For this review, take the finished solid that the model builds, in its own axes (mm). Coordinates: 2 decimals unless noted, no trailing zeros. Write each loop counter-clockwise with the first axis right and the second up, starting at its lowest first coordinate (ties: lowest second). Pieces come first, ordered by that corner, then holes. Notation, with made-up numbers: M -18,56.5 L 35,56.5 A16 cw 35,80.5 Z; hole C 79,47 d5. An arc over 180 degrees is marked long. Return JSON: item names as keys, results as strings.
```python
from build123d import *

# Parameters (mm, degrees)
SKETCH1_R = 25.4


with BuildPart() as part:
    # Sweep1: sweep along a curve in space
    with BuildLine() as sweep1_path:
        Line((0, 36.968559092, 0), (0, 36.968559092, -76.2))
        ThreePointArc((0, 36.968559092, -76.2), (0, 22.089583576, -112.121024484), (0, -13.831440908, -127))
        Line((0, -13.831440908, -127), (0, -217.031440908, -127))
        ThreePointArc((0, -217.031440908, -127), (0, -252.952465392, -112.121024484), (0, -267.831440908, -76.2))
        Line((0, -267.831440908, -76.2), (0, -267.831440908, -1.63913495))
        Line((0, -267.831440908, -1.63913495), (0, -267.831440908, 76.2))
        ThreePointArc((0, -267.831440908, 76.2), (0, -252.952465392, 112.121024484), (0, -217.031440908, 127))
        Line((0, -217.031440908, 127), (0, -13.831440908, 127))
        ThreePointArc((0, 36.968559092, 76.2), (0, 22.089583576, 112.121024484), (0, -13.831440908, 127))
        Line((0, 36.968559092, 0), (0, 36.968559092, 76.2))
    # Sketch1 → Sweep1 (sweep)
    with BuildSketch(Plane.XY):
        with Locations((0, 36.968559092)):
            Circle(SKETCH1_R)
    sweep(path=sweep1_path.line)


solid = part.part
```
1. We need section D-D (x = -19). State the section outline as (y, z) points, plus the area to 3 significant figures.
Checks:
{"outline": "M -284.69,-76.2 A67.66 ccw -217.03,-143.86 L -13.83,-143.86 A67.66 ccw 53.83,-76.2 L 53.83,76.2 A67.66 ccw -13.83,143.86 L -217.03,143.86 A67.66 ccw -284.69,76.2 Z; hole M -250.97,-76.2 A33.94 ccw -217.03,-110.14 L -13.83,-110.14 A33.94 ccw 20.11,-76.2 L 20.11,76.2 A33.94 ccw -13.83,110.14 L -217.03,110.14 A33.94 ccw -250.97,76.2 Z", "area": "34,700 mm2"}
2. Clearance check with flat-ended pins moving along their axes: pin 1 Ø5 at (x, z) = (-11.5, 75) entering from +Y; pin 2 Ø2 at (x, z) = (15.5, -63.5) entering from +Y; pin 3 Ø10 at (x, y) = (10, 17.5) entering from +Z. State where each tip first meets the part, or that it passes through.
Checks:
{"pin 1": "y = 60.72", "pin 2": "y = 57.82", "pin 3": "z = 146.28"}
3. Wall thickness on L1, parallel to Z at x = 2, y = -47.5; L2, parallel to Z at x = -18.5, y = -39; L3, parallel to Y at x = -18.5, z = -49: over which ranges is each line inside the solid? List them lowest first. Write a range as from..to.
Checks:
{"L1": "-152.32..-101.68, 101.68..152.32", "L2": "-144.4..-109.6, 109.6..144.4", "L3": "-285.24..-250.43, 19.56..54.37"}
4. We need section A-A (x = 0). State the section outline as (y, z) points, plus the area to 3 significant figures.
Checks:
{"outline": "M -293.23,-76.2 A76.2 ccw -217.03,-152.4 L -13.83,-152.4 A76.2 ccw 62.37,-76.2 L 62.37,76.2 A76.2 ccw -13.83,152.4 L -217.03,152.4 A76.2 ccw -293.23,76.2 Z; hole M -242.43,-76.2 A25.4 ccw -217.03,-101.6 L -13.83,-101.6 A25.4 ccw 11.57,-76.2 L 11.57,76.2 A25.4 ccw -13.83,101.6 L -217.03,101.6 A25.4 ccw -242.43,76.2 Z", "area": "52,300 mm2"}
5. We need section C-C (z = -2). State the section outline as (x, y) points, plus the area to 3 significant figures.
Checks:
{"outline": "C 0,-267.83 d50.8; C 0,36.97 d50.8", "area": "4,050 mm2"}
6. We need section B-B (y = -56.5). State the section outline as (x, z) points.
Checks:
{"outline": "C 0,-127 d50.8; C 0,127 d50.8"}
